from build123d import *

# Parameters (mm, degrees)
BASEHEAD_DEPTH      = 4.38
BOSS_EXTRUDE1_DEPTH = 5


with BuildPart() as part:
    # Sketch1 → BaseHead (new body)
    with BuildSketch(Plane(origin=(0, 0, 0), x_dir=(0, 0, -1), z_dir=(1, 0, 0))):
        Polygon((5, 2.886751346), (5, -2.886751346), (0, -5.773502692), (-5, -2.886751346), (-5, 2.886751346), (0, 5.773502692), align=None)
    extrude(amount=BASEHEAD_DEPTH)

    # BodySke → BaseBody (revolve)
    with BuildSketch(Plane.XY, mode=Mode.PRIVATE) as basebody_sk:
        Polygon((0, 0), (29.38, 0), (29.38, 2.4455), (28.8255, 3), (0, 3), align=None)
    revolve(basebody_sk.sketch.rotate(Axis((0, 0, 0), (1, 0, 0)), 90), axis=Axis((0, 0, 0), (1, 0, 0)))

    # Sketch3 → HeadChamfer (revolve, cut)
    with BuildSketch(Plane.XY):
        Polygon((0, 5), (3.333333333, 10.773502692), (3.333333333, 15.773502692), (-10, 15.773502692), (-10, 5), align=None)
    revolve(axis=Axis((0, 0, 0), (1, 0, 0)), mode=Mode.SUBTRACT)

    # Sketch4 → Boss-Extrude1 (add)
    with BuildSketch(Plane(origin=(25.38, 0, 0), x_dir=(0, 0, -1), z_dir=(1, 0, 0))):
        Polygon((0, 5.773502692), (-5, 2.886751346), (-5, -2.886751346), (0, -5.773502692), (5, -2.886751346), (5, 2.886751346), align=None)
    extrude(amount=-BOSS_EXTRUDE1_DEPTH)


solid = part.part
Source: CAD feature listing. Evaluate the final solid. Frame: model axes, mm. A direction names the side the tool comes from. Give positions to 0.01 mm unless a question says otherwise; leave off trailing zeros. Write each loop counter-clockwise with the first axis right and the second up, starting at its lowest first coordinate (ties: lowest second). Pieces come first, ordered by that corner, then holes. Notation, with made-up numbers: M 66,70.5 L 115,70.5 A27 cw 115,99.5 Z; hole C -28,67.25 d8. An arc over 180 degrees is marked long. Return JSON: item names as keys, results as strings. Group by question number.
1) Cut plane A-A, the plane x = 3.5. Output: boundary loops of the cut face in (y, z).
2) Set-up query: faces 1 (the face through (27.08, -0.9, 2.86)), 2 (the face through (20.38, -2.5, -2.2)), 3 (the face through (2.159, -4.35, 2.465)). Return all of +Z, -Z, +X, -X, +Y, -Y with unobstructed straight access to the full face (end or side cutting, diameter ignored); none if empty.
3) Pin query (flat end, axial travel): P1, Ø5, axis at x = 7, y = -0.5, coming from the -Z side; P2, Ø1.5, axis at x = 24.5, z = -2, coming from the -Y side; P3, Ø3, axis at x = 9, y = 3.5, coming from the +Z side. Return the tip coordinate at first contact, or that it passes through.
4) Pull-direction query (X, two-part tool) for faces 4 (the face through (22.915, 4.35, 2.465)), 5 (the face through (25.38, -2.5, -2.2)), 6 (the face through (4.38, -2.5, 2.2)), 7 (the face through (0.11, -5.19, 0.01)); classes: pulls with the +X half, pulls with the -X half, needs draft (parallel to the pull), parting line crosses it, or undercut.
5) Material intervals for line 1 along X through (y, z) = (-2, 3.75); line 2 along Y through (x, z) = (23.25, 2.5); line 3 along Y through (x, z) = (8, -2.5), sorted ascending. Write a range as [from, to].
6) Cut plane B-B, the plane x = 9.75. Output: boundary loops of the cut face in (y, z).
Recorded:
{
 "1": {"outline": "M -5.77,0 L -2.89,-5 L 2.89,-5 L 5.77,0 L 2.89,5 L -2.89,5 Z"},
 "2": {"face 1": "+X", "face 2": "none", "face 3": "+Z, +X, -X, -Y"},
 "3": {"P1": "stops at z = -3", "P2": "stops at y = -5.05", "P3": "stops at z = 2.24"},
 "4": {"face 4": "needs draft", "face 5": "pulls with the +X half", "face 6": "undercut", "face 7": "pulls with the -X half"},
 "5": {"line 1": "x = [0, 4.38], [20.38, 25.38]", "line 2": "y = [-4.33, 4.33]", "line 3": "y = [-1.66, 1.66]"},
 "6": {"outline": "C 0,0 d6"}
}
